For this review, take the finished solid that the model builds, in its own axes (mm). Face numbers are marked on the shaded views. A direction names the side the tool comes from. Coordinates: 2 decimals unless noted, no trailing zeros.
1. To check wall thickness, follow probe 1 along Z at (x, y) = (0, -9); probe 2 along Z at (x, y) = (0, -0.3); probe 3 along Y at (x, z) = (-2, -5.75). State the ranges of each line that lie inside material, in increasing order.
2. Machinability: for the marked faces 1 and 2, which of the approach directions +Z, -Z, +X, -X, +Y, -Y give a long, thin tool a straight path to every point of the face, cutting with its end or side? Answer none if there is none.
3. Clearance check with flat-ended pins moving along their axes: P1, Ø1.5, axis at x = 26.5, z = 3, coming from the -Y side; P2, Ø8, axis at x = 17, y = -4.5, coming from the -Z side; P3, Ø6, axis at x = -1, z = 0, coming from the +Y side; P4, Ø2, axis at x = 8, z = 5, coming from the +Y side. State where each tip first meets the part, or that it passes through.
4. Take a section at A-A, the plane z = 0. Count the separate pieces of the cut face and the enclosed holes in it, then the cut area to 3 significant figures.
5. Mouldability with a two-part tool opening along X and no side actions: class the marked faces 3, 4, 5 and 6 as pulls with the +X half, pulls with the -X half, needs draft (parallel to the pull), parting line crosses it, or undercut.
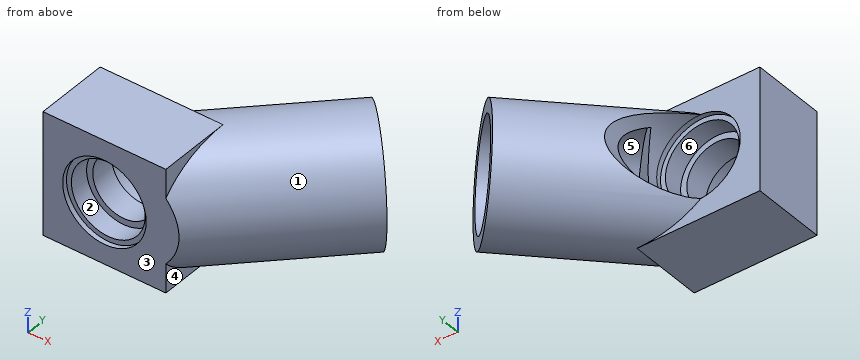
```python
from build123d import *

# Parameters (mm, degrees)
F0_W          = 20
F0_H          = 20
F1_DEPTH      = 12
F3_R          = 10
F4_DEPTH      = 20
F4_DEPTH_BACK = 9
F5_R          = 6.8
F6_DEPTH      = 0.8
F7_R          = 6.8
F8_DEPTH      = 0.8
F8_DEPTH_BACK = 25
F9_R          = 6
F10_DEPTH     = 3.2
F11_R         = 6
F12_DEPTH     = 3.2
F13_R         = 5
F14_DEPTH     = 4
F15_W         = 6.5863579512
F15_H         = 20
F16_DEPTH     = 25
F17_R         = 8
F18_DEPTH     = 21


with BuildPart() as f1:
    # F0 (on Front) → F1 (new body)
    with BuildSketch(Plane.XZ):
        Rectangle(F0_W, F0_H)
    extrude(amount=F1_DEPTH)

    # F3 (on face) → F4 (join, two sides)
    with BuildSketch(Plane(origin=(5, 5, 0), x_dir=(0.7071067812, -0.7071067812, 0), z_dir=(-0.7071067812, -0.7071067812, 0))) as f4_sk:
        with Locations((7.0710678119, 0)):
            Circle(F3_R)
    extrude(amount=-F4_DEPTH)
    extrude(f4_sk.sketch, amount=F4_DEPTH_BACK)

    # F5 (on face) → F6 (cut)
    with BuildSketch(Plane.XZ.offset(12)):
        Circle(F5_R)
    extrude(amount=-F6_DEPTH, mode=Mode.SUBTRACT)

    # F7 (on face) → F8 (cut, two sides)
    with BuildSketch(Plane(origin=(0, 0, 0), x_dir=(-1, 0, 0), z_dir=(0, 1, 0))) as f8_sk:
        Circle(F7_R)
    extrude(amount=-F8_DEPTH, mode=Mode.SUBTRACT)
    extrude(f8_sk.sketch, amount=F8_DEPTH_BACK, mode=Mode.SUBTRACT)

    # F9 (on face) → F10 (cut)
    with BuildSketch(Plane(origin=(0, -0.8, 0), x_dir=(-1, 0, 0), z_dir=(0, 1, 0))):
        Circle(F9_R)
    extrude(amount=-F10_DEPTH, mode=Mode.SUBTRACT)

    # F11 (on face) → F12 (cut)
    with BuildSketch(Plane.XZ.offset(11.2)):
        Circle(F11_R)
    extrude(amount=-F12_DEPTH, mode=Mode.SUBTRACT)

    # F13 (on face) → F14 (cut, through all)
    with BuildSketch(Plane.XZ.offset(8)):
        Circle(F13_R)
    extrude(amount=-F14_DEPTH, mode=Mode.SUBTRACT)

    # F15 (on Right) → F16 (cut)
    with BuildSketch(Plane.YZ):
        with Locations((-15.2931789756, 0)):
            Rectangle(F15_W, F15_H)
    extrude(amount=F16_DEPTH, mode=Mode.SUBTRACT)

    # F17 (on face) → F18 (cut)
    with BuildSketch(Plane(origin=(19.1421356237, 19.1421356237, 0), x_dir=(-0.7071067812, 0.7071067812, 0), z_dir=(0.7071067812, 0.7071067812, 0))):
        with Locations((-7.0710678119, 0)):
            Circle(F17_R)
    extrude(amount=-F18_DEPTH, mode=Mode.SUBTRACT)


solid = f1.part
```
Results list:
1. probe 1: z = -10 to -6, 6 to 10
1. probe 2: z = -10 to -6.8, 6.8 to 10
1. probe 3: y = -11.2 to -0.8
2. face 1: none
2. face 2: -Y
3. P1: stops at y = 2.2
3. P2: stops at z = -9.11
3. P3: passes through
3. P4: stops at y = 11.5
4. separate pieces: 3
4. enclosed holes: 0
4. area: 213 mm2
5. face 3: needs draft
5. face 4: pulls with the +X half
5. face 5: undercut
5. face 6: undercut
